Job drawing, mm, ordinate dimensions from the low corner. One solid piece. Round coordinates to 2 decimals unless told otherwise and drop trailing zeros.
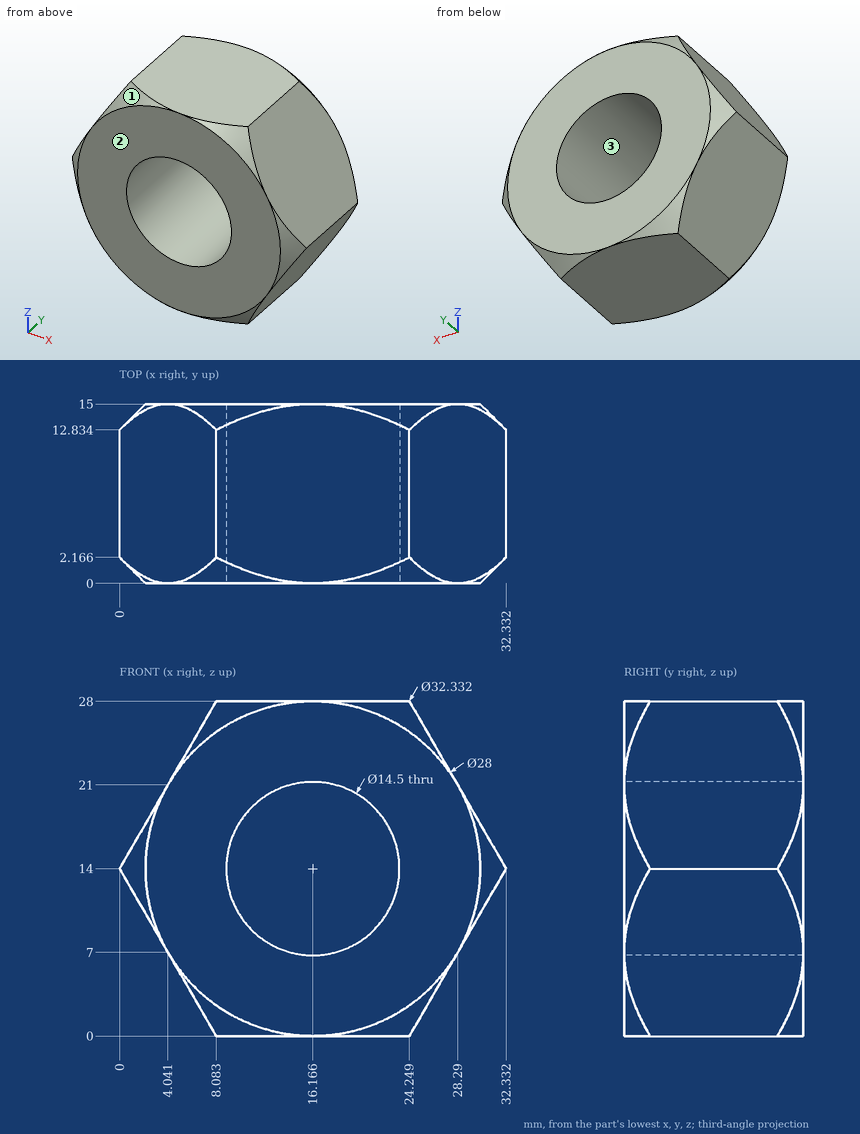
Item 1: Probe line 1 (Z direction, x = 16, y = 6.75); line 2 (X direction, y = 11, z = 10.5) (1 decimal); line 3 (X direction, y = 12, z = 16) (1 decimal). List the from-to ranges inside material, lowest first.
Answers follow:
line 1: z = 0 to 6.75, 21.25 to 28
line 2: x = 2 to 9.8, 22.5 to 30.3
line 3: x = 1.2 to 9.2, 23.1 to 31.2
Item 2: Flat gauge pins, fed straight in: P1, Ø4, axis at x = 19.5, z = 16, coming from the -Y side; P2, Ø1, axis at y = 8.5, z = 16.5, coming from the +X side; P3, Ø3, axis at x = 4.5, z = 24.5, coming from the +Y side (1 decimal). Where does each tip first touch, or does it go through?
Answers follow:
P1: passes through
P2: stops at x = 31.18
P3: stops at y = 14.8
Item 3: Two-plate mould, pull along X, no slides. Class the marked faces 1, 2 and 3: released by +X, released by -X, zero draft, split by the parting line, or undercut.
Answers follow:
face 1: released by -X
face 2: zero draft
face 3: undercut
